Geometry: final body of the model. Coordinates: model frame, mm. A direction names the side the tool comes from. Give positions to 0.01 mm unless a question says otherwise; leave off trailing zeros. Write each loop counter-clockwise with the first axis right and the second up, starting at its lowest first coordinate (ties: lowest second). Pieces come first, ordered by that corner, then holes.
```python
from build123d import *

# Parameters (mm, degrees)
F0_R         = 11
F0_R_2       = 6
F1_DEPTH     = 25
F2_R         = 11
F3_DEPTH     = 5
F5_DEPTH     = 12.5
F7_DEPTH     = 5
F8_R         = 10
F9_T4_ANGLE  = 90
F9_S5_R      = 18.3546430422
F9_T6_DEPTH  = 14
F9_T10_ANGLE = 270
F9_S11_R     = 18.3546430422
F9_T12_DEPTH = 26
F9_T16_ANGLE = 270
F9_S17_R     = 18.3546430422
F9_T18_DEPTH = 26
F9_T22_ANGLE = 270
F9_S23_R     = 18.3546430422
F9_T24_DEPTH = 26
F9_T28_ANGLE = 270
F9_S29_R     = 18.3546430422
F9_T30_DEPTH = 26
F9_T34_ANGLE = 90
F9_S35_R     = 18.3546430422
F9_T36_DEPTH = 14
F10_R        = 6
F11_DEPTH    = 30
F12_R        = 2.5
F13_DEPTH    = 5.001


# Not quite as in the source:
# - a fillet or chamfer that OpenCascade refuses, or shapes differently, is made with other operations: its cross-section is extruded or revolved along the edge and cut away or added


with BuildPart() as f1:
    # F0 (on Front) → F1 (new body, symmetric)
    with BuildSketch(Plane.XZ):
        Circle(F0_R)
        Circle(F0_R_2, mode=Mode.SUBTRACT)
    extrude(amount=F1_DEPTH, both=True)

    # F2 (on face) → F3 (join)
    with BuildSketch(Plane(origin=(0, 25, 0), x_dir=(-1, 0, 0), z_dir=(0, 1, 0))):
        Circle(F2_R)
    extrude(amount=F3_DEPTH)

    # F4 (on Front) → F5 (join, symmetric)
    with BuildSketch(Plane.XZ):
        with BuildLine():
            ThreePointArc((-17.8147200495, 0), (-10.6296195649, -8.2892337781), (0, -11))
            ThreePointArc((0, -11), (10.6296195649, -8.2892337781), (17.8147200495, 0))
            Line((17.8147200495, 0), (17.8147200495, 90))
            Line((17.8147200495, 90), (-17.8147200495, 90))
            Line((-17.8147200495, 90), (-17.8147200495, 0))
        make_face()
        with BuildLine():
            ThreePointArc((0, -11), (-7.7781745931, 7.7781745931), (11, 0))
            ThreePointArc((11, 0), (7.7781745931, -7.7781745931), (0, -11))
        make_face(mode=Mode.SUBTRACT)
        with BuildLine():
            ThreePointArc((0, -11), (7.7781745931, -7.7781745931), (11, 0))
            ThreePointArc((11, 0), (-7.7781745931, 7.7781745931), (0, -11))
        make_face()
    extrude(amount=F5_DEPTH, both=True)

    # F6 (on face) → F7 (join)
    with BuildSketch(Plane.XY.offset(90)):
        Polygon((17.8147200495, -52.5), (17.8147200495, -12.5), (17.8147200495, 12.5), (17.8147200495, 52.5), (-17.8147200495, 52.5), (-17.8147200495, 12.5), (-17.8147200495, -12.5), (-17.8147200495, -52.5), align=None)
    extrude(amount=F7_DEPTH)

    # F8
    f8_edges = [f1.edges().sort_by_distance(p)[0] for p in [
        (0, -12.5, 90),
        (0, 12.5, 90),
    ]]
    fillet(f8_edges, radius=F8_R)

    # F9: fillet of radius 5 on 4 edges, made by hand


with BuildPart() as f9_tool2:
    # F9_s3 → F9_t4 (revolve)
    with BuildSketch(Plane.YZ):
        with BuildLine():
            ThreePointArc((-12.5, -16), (-13.9644660941, -12.4644660941), (-17.5, -11))
            Line((-17.5, -11), (-12.5, -11))
            Line((-12.5, -11), (-12.5, -16))
        make_face()
    revolve(axis=Axis((0, -12.5, 0), (0, -1, 0)), revolution_arc=F9_T4_ANGLE)

    # F9_s5 → F9_t6 (intersect, symmetric)
    with BuildSketch(Plane.XZ.offset(16.8)):
        with Locations((0.9864220241, 7.3281175465)):
            Circle(F9_S5_R)
    extrude(amount=F9_T6_DEPTH, both=True, mode=Mode.INTERSECT)


with BuildPart() as f1_1:
    add(f1.part)

    # F9_t1: union F9_tool2
    add(f9_tool2.part)


with BuildPart() as f9_tool8:
    # F9_s9 → F9_t10 (revolve)
    with BuildSketch(Plane.XY):
        with BuildLine():
            ThreePointArc((16, -12.5), (12.4644660941, -13.9644660941), (11, -17.5))
            Line((11, -17.5), (11, -12.5))
            Line((11, -12.5), (16, -12.5))
        make_face()
    revolve(axis=Axis((0, -12.5, 0), (0, -1, 0)), revolution_arc=F9_T10_ANGLE)

    # F9_s11 → F9_t12 (intersect, symmetric)
    with BuildSketch(Plane.XZ.offset(16.8)):
        with Locations((0.9864220241, 7.3281175465)):
            Circle(F9_S11_R)
    extrude(amount=F9_T12_DEPTH, both=True, mode=Mode.INTERSECT)


with BuildPart() as f1_2:
    add(f1_1.part)

    # F9_t7: union F9_tool8
    add(f9_tool8.part)


with BuildPart() as f9_tool14:
    # F9_s15 → F9_t16 (revolve)
    with BuildSketch(Plane.XY):
        with BuildLine():
            ThreePointArc((16, -12.5), (12.4644660941, -13.9644660941), (11, -17.5))
            Line((11, -17.5), (11, -12.5))
            Line((11, -12.5), (16, -12.5))
        make_face()
    revolve(axis=Axis((0, -12.5, 0), (0, -1, 0)), revolution_arc=F9_T16_ANGLE)

    # F9_s17 → F9_t18 (intersect, symmetric)
    with BuildSketch(Plane.XZ.offset(16.8)):
        with Locations((-0.9864220241, 7.3281175465)):
            Circle(F9_S17_R)
    extrude(amount=F9_T18_DEPTH, both=True, mode=Mode.INTERSECT)


with BuildPart() as f1_3:
    add(f1_2.part)

    # F9_t13: union F9_tool14
    add(f9_tool14.part)


with BuildPart() as f9_tool20:
    # F9_s21 → F9_t22 (revolve)
    with BuildSketch(Plane.XY):
        with BuildLine():
            ThreePointArc((16, 12.5), (12.4644660941, 13.9644660941), (11, 17.5))
            Line((11, 17.5), (11, 12.5))
            Line((11, 12.5), (16, 12.5))
        make_face()
    revolve(axis=Axis((0, 12.5, 0), (0, -1, 0)), revolution_arc=F9_T22_ANGLE)

    # F9_s23 → F9_t24 (intersect, symmetric)
    with BuildSketch(Plane.XZ.offset(-16.8)):
        with Locations((0.9864220241, 7.3281175465)):
            Circle(F9_S23_R)
    extrude(amount=F9_T24_DEPTH, both=True, mode=Mode.INTERSECT)


with BuildPart() as f1_4:
    add(f1_3.part)

    # F9_t19: union F9_tool20
    add(f9_tool20.part)


with BuildPart() as f9_tool26:
    # F9_s27 → F9_t28 (revolve)
    with BuildSketch(Plane.XY):
        with BuildLine():
            ThreePointArc((16, 12.5), (12.4644660941, 13.9644660941), (11, 17.5))
            Line((11, 17.5), (11, 12.5))
            Line((11, 12.5), (16, 12.5))
        make_face()
    revolve(axis=Axis((0, 12.5, 0), (0, -1, 0)), revolution_arc=F9_T28_ANGLE)

    # F9_s29 → F9_t30 (intersect, symmetric)
    with BuildSketch(Plane.XZ.offset(-16.8)):
        with Locations((-0.9864220241, 7.3281175465)):
            Circle(F9_S29_R)
    extrude(amount=F9_T30_DEPTH, both=True, mode=Mode.INTERSECT)


with BuildPart() as f1_5:
    add(f1_4.part)

    # F9_t25: union F9_tool26
    add(f9_tool26.part)


with BuildPart() as f9_tool32:
    # F9_s33 → F9_t34 (revolve)
    with BuildSketch(Plane.YZ):
        with BuildLine():
            ThreePointArc((12.5, -16), (13.9644660941, -12.4644660941), (17.5, -11))
            Line((17.5, -11), (12.5, -11))
            Line((12.5, -11), (12.5, -16))
        make_face()
    revolve(axis=Axis((0, 12.5, 0), (0, -1, 0)), revolution_arc=F9_T34_ANGLE)

    # F9_s35 → F9_t36 (intersect, symmetric)
    with BuildSketch(Plane.XZ.offset(-16.8)):
        with Locations((0.9864220241, 7.3281175465)):
            Circle(F9_S35_R)
    extrude(amount=F9_T36_DEPTH, both=True, mode=Mode.INTERSECT)


with BuildPart() as f1_6:
    add(f1_5.part)

    # F9_t31: union F9_tool32
    add(f9_tool32.part)

    # F10 (on face) → F11 (cut)
    with BuildSketch(Plane.XZ.offset(12.5)):
        Circle(F10_R)
    extrude(amount=-F11_DEPTH, mode=Mode.SUBTRACT)

    # F12 (on face) → F13 (cut, through all)
    with BuildSketch(Plane(origin=(0, 0, 90), x_dir=(1, 0, 0), z_dir=(0, 0, -1))):
        with Locations((-11.8147200495, 46.5)):
            Circle(F12_R)
        with Locations((11.8147200495, 46.5)):
            Circle(F12_R)
        with Locations((-11.8147200495, -46.5)):
            Circle(F12_R)
        with Locations((11.8147200495, -46.5)):
            Circle(F12_R)
    extrude(amount=-F13_DEPTH, mode=Mode.SUBTRACT)


solid = f1_6.part
```
Item 1: Pull-direction query (X, two-part tool) for faces 1 (the face through (-2.38, -21.3, -10.74)), 2 (the face through (0, -37, 90)), 3 (the face through (0, 25, 0)), 4 (the face through (11.27, 48.94, 92.46)); classes: +X half, -X half, draft (parallel to the pull), parting line (faces both ways), or undercut.
Found:
face 1: parting line
face 2: draft
face 3: undercut
face 4: undercut
Item 2: Section D-D, the plane z = 86.5. Return the cut outline in (x, y).
Found:
outline: (-17.81, -14.9) - (17.81, -14.9) - (17.81, 14.9) - (-17.81, 14.9) - close
Item 3: Section A-A, the plane y = -46.5. Return the cut outline in (x, z), plus the area to 3 significant figures.
Found:
outline: (-17.81, 90) - (-14.31, 90) - (-14.31, 95) - (-17.81, 95) - close; (-9.31, 90) - (9.31, 90) - (9.31, 95) - (-9.31, 95) - close; (14.31, 90) - (17.81, 90) - (17.81, 95) - (14.31, 95) - close
area: 128 mm2
Item 4: Line query: L1, parallel to X at y = -46.5, z = 92.65; L2, parallel to X at y = -22, z = 0; L3, parallel to Z at x = 0, y = 19. Output: solid intervals per line, ascending.
Found:
L1: x = -17.81 to -14.31, -9.31 to 9.31, 14.31 to 17.81
L2: x = -11 to -6, 6 to 11
L3: z = -11 to -6, 6 to 11, 89.37 to 95
Item 5: Section B-B, the plane y = 14. Return the cut outline in (x, z).
Found:
outline: (-17.81, 85.27) - (17.81, 85.27) - (17.81, 95) - (-17.81, 95) - close; (-7.71, -9.75) arc R18.35 ccw to (0, -11) arc R18.35 ccw to (7.71, -9.75) arc R12.43 ccw (long way) to start; hole circle Ø12 at (0, 0)
Item 6: Section C-C, the plane y = 39. Return the cut outline in (x, z), plus the area to 3 significant figures.
Found:
outline: (-17.81, 90) - (17.81, 90) - (17.81, 95) - (-17.81, 95) - close
area: 178 mm2
Item 7: Reachability of faces 5 (the face through (-0.25, -15.51, 87.15)), 6 (the face through (5, -25, -5)), 7 (the face through (0, 38, 90)) from +Z, -Z, +X, -X, +Y, -Y: full face, straight path, thin tool, end or side. Return the list, or none.
Found:
face 5: +X, -X, -Y
face 6: -Z, +X, -X, -Y
face 7: +X, -X, +Y
Item 8: Pin query (flat end, axial travel): pin 1 Ø6.5 at (x, y) = (11.81, 46.5) entering from -Z; pin 2 Ø11 at (x, z) = (0, 0) entering from +Y; pin 3 Ø6 at (x, y) = (11, 3.5) entering from -Z; pin 4 Ø3 at (x, y) = (11.81, -46.5) entering from +Z. Return the tip coordinate at first contact, or that it passes through.
Found:
pin 1: stops at z = 90
pin 2: stops at y = 30
pin 3: stops at z = -9.63
pin 4: passes through
